Could you check a few things on this drawing? It's one solid part, dimensions in mm from its lowest x, y, z. A direction names the side the tool comes from. Give positions to 0.01 mm unless a question says otherwise; leave off trailing zeros. Loops run counter-clockwise (first coordinate to the right, second up) from the corner with the lowest first, then second, coordinate; pieces in that order, holes last. Notation, with made-up numbers: (-39, 29) - (-8, 29) arc R10 cw to (-8, 33) - close; hole circle Ø1 at (-38.75, 42.25). An arc over 180 degrees is marked (long way). Return JSON: item names as keys, results as strings. Group by question number.
(1) If we mould it in two halves opening along Y, with no side actions, what happens to the marked faces 1, 2, 3 and 4? For each: released by +Y, released by -Y, zero draft, split by the parting line, or undercut.
(2) I need wall thicknesses on probe 1 along Y at (x, z) = (153, 131.5); probe 2 along Z at (x, y) = (282, 316); probe 3 along X at (y, z) = (292.5, 324.5). Which ranges of each line are inside material? Lowest first, please. Write a range as [from, to].
(3) If we section it at B-B (x = 153): Please give me the cut outline in (y, z), then the cut area to 3 significant figures.
(4) For P1, Ø12, axis at x = 402.5, z = 461, coming from the +Y side; P2, Ø1, axis at x = 384, z = 171, coming from the +Y side; P3, Ø6, axis at y = 210, z = 473, coming from the -X side, each with a flat end and sliding along its axis, tell me the tip position at first contact or that it passes through.
(5) If we section it at D-D (z = 442): Please give me the cut outline in (x, y), then the cut area to 3 significant figures.
(6) If we section it at A-A (y = 198): Please give me the cut outline in (x, z).
(7) If we section it at C-C (z = 229.5): Please give me the cut outline in (x, y).
(8) On a 3-axis mill with a long thin cutter (end or side, diameter ignored), from which of +Z, -Z, +X, -X, +Y, -Y can I reach the whole of each face in a straight line? I mean the marked faces 5 and 6. Say none if no direction works.
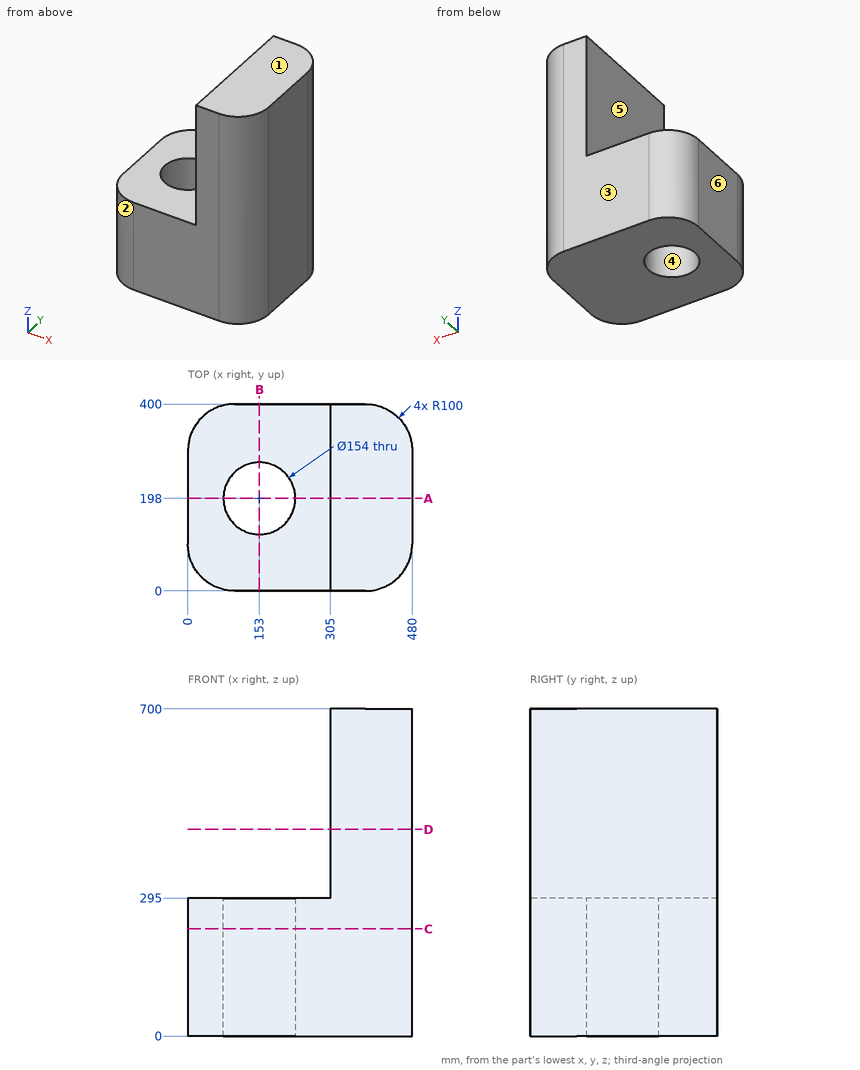
Values:
{
 "1": {"face 1": "zero draft", "face 2": "released by -Y", "face 3": "released by +Y", "face 4": "undercut"},
 "2": {"probe 1": "[0, 121], [275, 400]", "probe 2": "[0, 295]", "probe 3": "[305, 480]"},
 "3": {"outline": "(0, 0) - (121, 0) - (121, 295) - (0, 295) - close; (275, 0) - (400, 0) - (400, 295) - (275, 295) - close", "area": "72,600 mm2"},
 "4": {"P1": "y = 398.63", "P2": "y = 399.94", "P3": "x = 305"},
 "5": {"outline": "(305, 0) - (380, 0) arc R100 ccw to (480, 100) - (480, 300) arc R100 ccw to (380, 400) - (305, 400) - close", "area": "65,700 mm2"},
 "6": {"outline": "(0, 0) - (76, 0) - (76, 295) - (0, 295) - close; (230, 0) - (480, 0) - (480, 700) - (305, 700) - (305, 295) - (230, 295) - close"},
 "7": {"outline": "(0, 100) arc R100 ccw to (100, 0) - (380, 0) arc R100 ccw to (480, 100) - (480, 300) arc R100 ccw to (380, 400) - (100, 400) arc R100 ccw to (0, 300) - close; hole circle Ø154 at (153, 198)"},
 "8": {"face 5": "+Z, -X, +Y, -Y", "face 6": "+Z, -Z, -X, +Y, -Y"}
}
